Could you check a few things on this model? Use its own coordinates, in mm. Face numbers are marked on the shaded views. A direction names the side the tool comes from. Round coordinates to 2 decimals unless told otherwise and drop trailing zeros. Order: outer loops, then holes, each group sorted by start corner. A loop starts at its lowest first (then second) coordinate and runs counter-clockwise, first axis right, second up. Notation, with made-up numbers: (19, -19.5) - (41, -19.5) arc R9 cw to (41, -8.5) - close; hole circle Ø9 at (-16.5, -31). An arc over 180 degrees is marked (long way). Use one line per item in the form item = value.
from build123d import *

# Parameters (mm, degrees)
SKETCH2_W               = 457.2
SKETCH2_H               = 609.6
SKETCH2_W_2             = 76.2
SKETCH2_H_2             = 25.4
BOSS_EXTRUDE1_DEPTH     = 17.78
SKETCH3_W               = 76.2
SKETCH3_H               = 25.4
BOSS_EXTRUDE2_DEPTH     = 116.586
SKETCH3_2_W             = 76.2
SKETCH3_2_H             = 25.4
BOSS_EXTRUDE3_DEPTH     = 17.78
CUT_EXTRUDE1_DEPTH      = 254
CUT_EXTRUDE1_DEPTH_BACK = 254
SKETCH4_R               = 12.7


with BuildPart() as part:
    # Sketch2 → Boss-Extrude1 (new body)
    with BuildSketch(Plane(origin=(0, 0, 0), x_dir=(1, 0, 0), z_dir=(0, 1, 0))):
        Rectangle(SKETCH2_W, SKETCH2_H)
        with Locations((-177.8, 0)):
            Rectangle(SKETCH2_W_2, SKETCH2_H_2, mode=Mode.SUBTRACT)
    extrude(amount=-BOSS_EXTRUDE1_DEPTH)



with BuildPart() as body_2:
    # Sketch3 → Boss-Extrude2 (new body)
    with BuildSketch(Plane(origin=(0, 0, 0), x_dir=(1, 0, 0), z_dir=(0, 1, 0))):
        with Locations((-177.8, 0)):
            Rectangle(SKETCH3_W, SKETCH3_H)
    extrude(amount=BOSS_EXTRUDE2_DEPTH)


with BuildPart() as part_1:
    add(part.part)

    add(body_2.part)  # Boss-Extrude3 merges body 2
    # Sketch3_2 → Boss-Extrude3 (add)
    with BuildSketch(Plane(origin=(0, 0, 0), x_dir=(1, 0, 0), z_dir=(0, 1, 0))):
        with Locations((-177.8, 0)):
            Rectangle(SKETCH3_2_W, SKETCH3_2_H)
    extrude(amount=-BOSS_EXTRUDE3_DEPTH)

    # Sketch4 → Cut-Extrude1 (cut, two sides: drawn at the far end of the back side and taken through both)
    with BuildSketch(Plane.XY.offset(-CUT_EXTRUDE1_DEPTH_BACK)):
        with Locations(Location((-177.8, 91.186, 0), (0, 0, 180))):
            Circle(SKETCH4_R)
    extrude(amount=CUT_EXTRUDE1_DEPTH + CUT_EXTRUDE1_DEPTH_BACK, mode=Mode.SUBTRACT)


solid = part_1.part
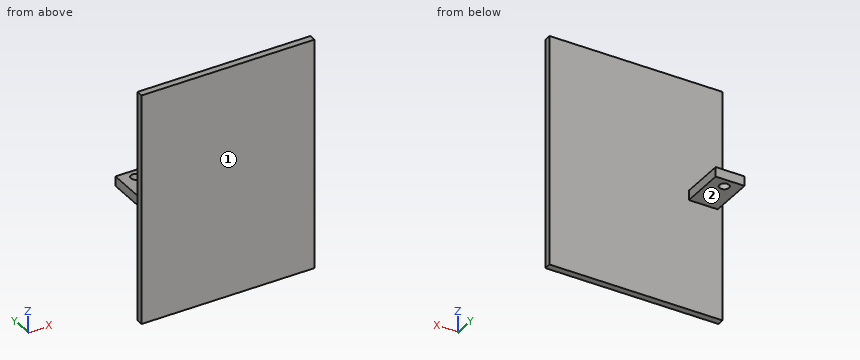
Item 1: Imagine slicing it at B-B on x = 75.5. Please give me the cut outline in (y, z), plus the area to 3 significant figures.
Found:
outline = (-17.78, -304.8) - (0, -304.8) - (0, 304.8) - (-17.78, 304.8) - close
area = 10,800 mm2
Item 2: For the marked faces 1 and 2, which set-ups out of +Z, -Z, +X, -X, +Y, -Y let a thin tool reach every point of the face, with its end or its side?
Found:
face_1 = +Z, -Z, +X, -X, -Y
face_2 = -Z, +X, -X, +Y
Item 3: Imagine slicing it at A-A on x = -177.8. Please give me the cut outline in (y, z).
Found:
outline = (-17.78, -304.8) - (0, -304.8) - (0, -12.7) - (78.49, -12.7) - (78.49, 12.7) - (0, 12.7) - (0, 304.8) - (-17.78, 304.8) - close; (103.89, -12.7) - (116.59, -12.7) - (116.59, 12.7) - (103.89, 12.7) - close
Item 4: I need wall thicknesses on L1, parallel to Y at x = -177.8, z = 5.5; L2, parallel to X at y = 1, z = -11.5; L3, parallel to Y at x = -197, z = -40.5. Which ranges of each line are inside material? Lowest first, please.
Found:
L1 = -17.78 to 78.49, 103.89 to 116.59
L2 = -215.9 to -139.7
L3 = -17.78 to 0
Item 5: Will these pins go through, and if not, where does the flat tip stop? P1, Ø20.5, axis at x = -177.8, y = 91.186, coming from the -Z side; P2, Ø6, axis at x = -22, z = 240.5, coming from the +Y side; P3, Ø20.5, axis at y = 70, z = -6, coming from the -X side; P4, Ø3, axis at y = 7.5, z = 13, coming from the +X side.
Found:
P1 = through
P2 = 0
P3 = -215.9
P4 = -139.7
Item 6: Imagine slicing it at C-C on y = 64.5. Please give me the cut outline in (x, z), plus the area to 3 significant figures.
Found:
outline = (-215.9, -12.7) - (-139.7, -12.7) - (-139.7, 12.7) - (-215.9, 12.7) - close
area = 1,940 mm2
